The drawing under review shows one solid part. Ordinate dimensions are in mm from its lowest x, y, z. Coordinates: 2 decimals unless noted, no trailing zeros. Order: outer loops, then holes, each group sorted by start corner. A loop starts at its lowest first (then second) coordinate and runs counter-clockwise, first axis right, second up.
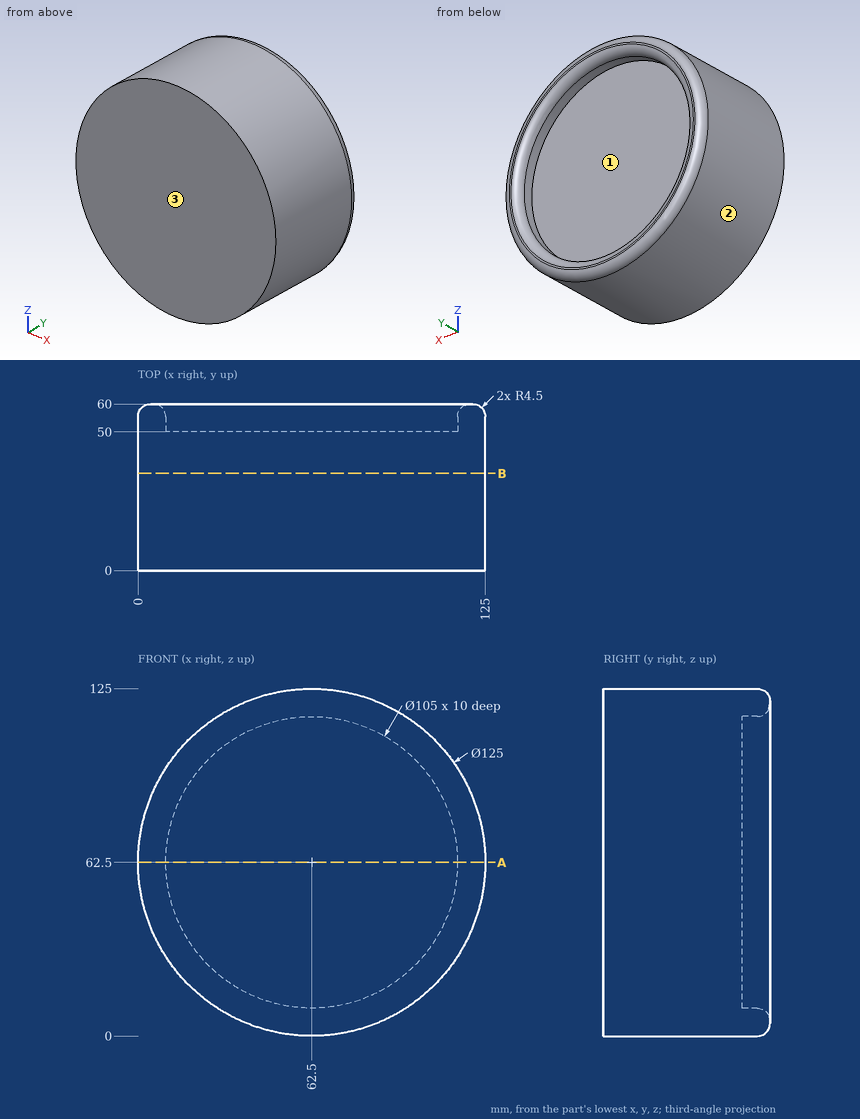
1. Clearance check with flat-ended pins moving along their axes: pin 1 Ø1.5 at (x, y) = (76, 21.5) entering from -Z; pin 2 Ø2 at (x, z) = (37.5, 33) entering from +Y; pin 3 Ø8 at (y, z) = (35.5, 54) entering from +X; pin 4 Ø6 at (x, z) = (47, 34.5) entering from -Y. State where each tip first meets the part, or that it passes through.
Answer below:
pin 1: stops at z = 1.31
pin 2: stops at y = 50
pin 3: stops at x = 124.84
pin 4: stops at y = 0
2. The part is to be moulded in two halves that separate along Z. For the marked faces 1, 2 and 3, say which applies: +Z half, -Z half, draft (parallel to the pull), parting line (faces both ways), or undercut.
Answer below:
face 1: undercut
face 2: parting line
face 3: draft
3. Take a section at A-A, the plane z = 62.5. Give the boundary of the cut face in (x, y).
Answer below:
outline: (0, 0) - (125, 0) - (125, 55.5) arc R4.5 ccw to (120.5, 60) - (119.5, 60) arc R4.5 ccw to (115, 55.5) - (115, 50) - (10, 50) - (10, 55.5) arc R4.5 ccw to (5.5, 60) - (4.5, 60) arc R4.5 ccw to (0, 55.5) - close
4. Take a section at B-B, the plane y = 35. Give the boundary of the cut face in (x, z), plus the area to 3 significant figures.
Answer below:
outline: circle Ø125 at (62.5, 62.5)
area: 12,300 mm2
5. To check wall thickness, follow L1, parallel to Z at x = 64, y = 50.5; L2, parallel to X at y = 51.6, z = 62.5; L3, parallel to Y at x = 93, z = 64.5. State the ranges of each line that lie inside material, in increasing order.
Answer below:
L1: z = 0.02 to 10.02, 114.98 to 124.98
L2: x = 0 to 10, 115 to 125
L3: y = 0 to 50
